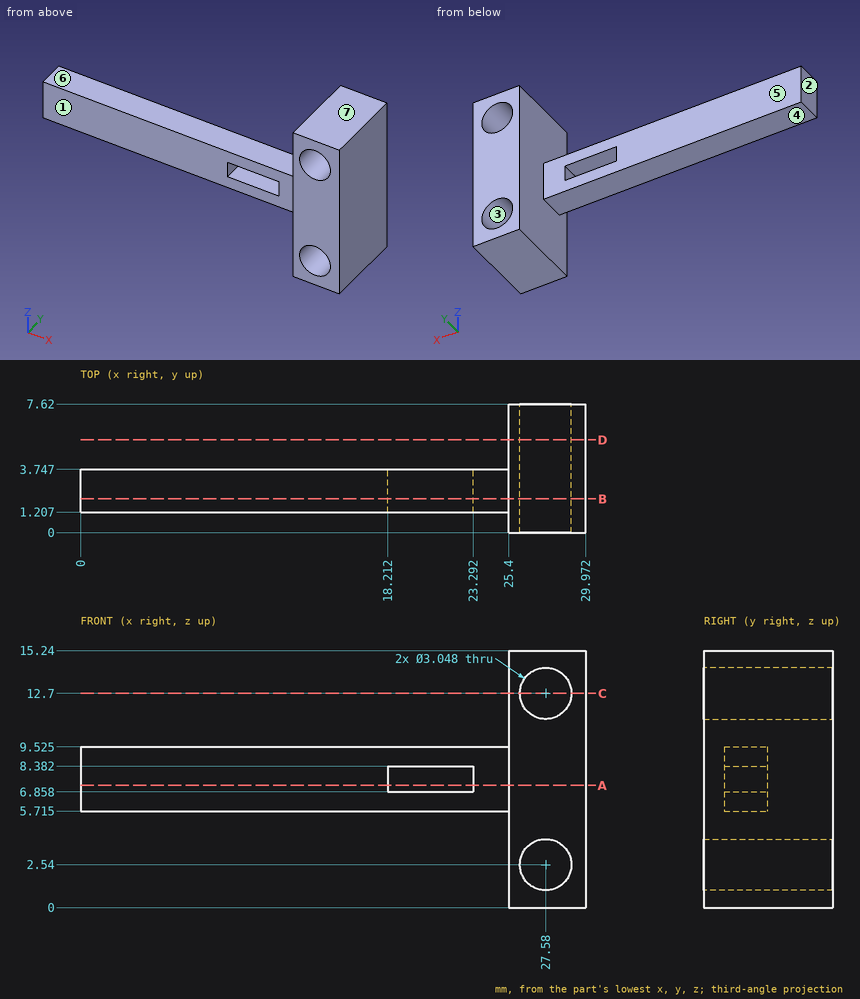
Answer from the drawing. Dimensions are ordinates in mm from the lowest x, y and z of the part. A direction names the side the tool comes from. Coordinates: 2 decimals unless noted, no trailing zeros. Write each loop counter-clockwise with the first axis right and the second up, starting at its lowest first coordinate (ties: lowest second). Pieces come first, ordered by that corner, then holes. Notation, with made-up numbers: M -11.5,-12 L 41.5,-12 A10 ccw 41.5,-6 Z; hole C 30.5,23.5 d11. An arc over 180 degrees is marked long. Use a Markdown table: item, result.
Q1. The part is cut by section B-B, the plane y = 2. Write down the section's boundary in (x, z) (1 decimal), then the cut area to 3 significant figures.
Answer block:
| item | result |
|---|---|
| outline | M 0,5.7 L 25.4,5.7 L 25.4,0 L 30,0 L 30,15.2 L 25.4,15.2 L 25.4,9.5 L 0,9.5 Z; hole M 18.2,6.9 L 23.3,6.9 L 23.3,8.4 L 18.2,8.4 Z; hole C 27.6,2.5 d3; hole C 27.6,12.7 d3 |
| area | 144 mm2 |
Q2. The part is cut by section A-A, the plane z = 7.25. Write down the section's boundary in (x, y).
Answer block:
| item | result |
|---|---|
| outline | M 0,1.21 L 18.21,1.21 L 18.21,3.75 L 0,3.75 Z; M 23.29,1.21 L 25.4,1.21 L 25.4,0 L 29.97,0 L 29.97,7.62 L 25.4,7.62 L 25.4,3.75 L 23.29,3.75 Z |
Q3. The part is cut by section D-D, the plane y = 5.5. Write down the section's boundary in (x, z).
Answer block:
| item | result |
|---|---|
| outline | M 25.4,0 L 29.97,0 L 29.97,15.24 L 25.4,15.24 Z; hole C 27.58,2.54 d3.05; hole C 27.58,12.7 d3.05 |
Q4. The part is cut by section C-C, the plane z = 12.7. Write down the section's boundary in (x, y), then the cut area to 3 significant figures.
Answer block:
| item | result |
|---|---|
| outline | M 25.4,0 L 26.06,0 L 26.06,7.62 L 25.4,7.62 Z; M 29.1,0 L 29.97,0 L 29.97,7.62 L 29.1,7.62 Z |
| area | 11.6 mm2 |
Q5. Which of the six approach directions +Z, -Z, +X, -X, +Y, -Y give full straight-line access (tool end or side, diameter ignored) to the marked faces 4, 5, 6 and 7?
Answer block:
| item | result |
|---|---|
| face 4 | -Z, -X, +Y, -Y |
| face 5 | +Z, -Z, -X, +Y |
| face 6 | +Z, -X, +Y, -Y |
| face 7 | +Z, +X, -X, +Y, -Y |
Q6. Determine the mould class of the marked faces 1, 2 and 3 for opening direction X: released by +X, released by -X, zero draft, split by the parting line, or undercut.
Answer block:
| item | result |
|---|---|
| face 1 | zero draft |
| face 2 | released by -X |
| face 3 | undercut |
Q7. Each of these flat-tipped pins is pushed along its axis until it touches: pin 1 Ø2 at (x, y) = (21, 2) entering from -Z (3 decimals); pin 2 Ø4 at (x, z) = (13.5, 7.5) entering from +Y; pin 3 Ø1.8 at (x, z) = (27.58, 12.7) entering from -Y; pin 4 Ø2 at (x, y) = (20.5, 3) entering from +Z (3 decimals). Where does it stop, or does it pass through?
Answer block:
| item | result |
|---|---|
| pin 1 | stops at z = 5.715 |
| pin 2 | stops at y = 3.75 |
| pin 3 | passes through |
| pin 4 | stops at z = 9.525 |
Q8. Straight lines are drawn through the part: L1, parallel to X at y = 6, z = 2.54; L2, parallel to X at y = 3.5, z = 7; L3, parallel to X at y = 5, z = 9.5. For each, find the intervals that lie inside material, in ascending order. Write a range as [from, to].
Answer block:
| item | result |
|---|---|
| L1 | x = [25.4, 26.06], [29.1, 29.97] |
| L2 | x = [0, 18.21], [23.29, 29.97] |
| L3 | x = [25.4, 29.97] |
